Can you work these out from the drawing? Everything is in mm from the part's minimum corner. Round coordinates to 2 decimals unless told otherwise and drop trailing zeros. Order: outer loops, then holes, each group sorted by start corner. A loop starts at its lowest first (then second) coordinate and runs counter-clockwise, first axis right, second up. Notation, with made-up numbers: (-1.75, -39.75) -> (53.25, -39.75) arc R15 cw to (53.25, -11.75) -> close; hole circle Ø10 at (-18.75, 35.5). An arc over 180 degrees is marked (long way). One line per item, written item: value.
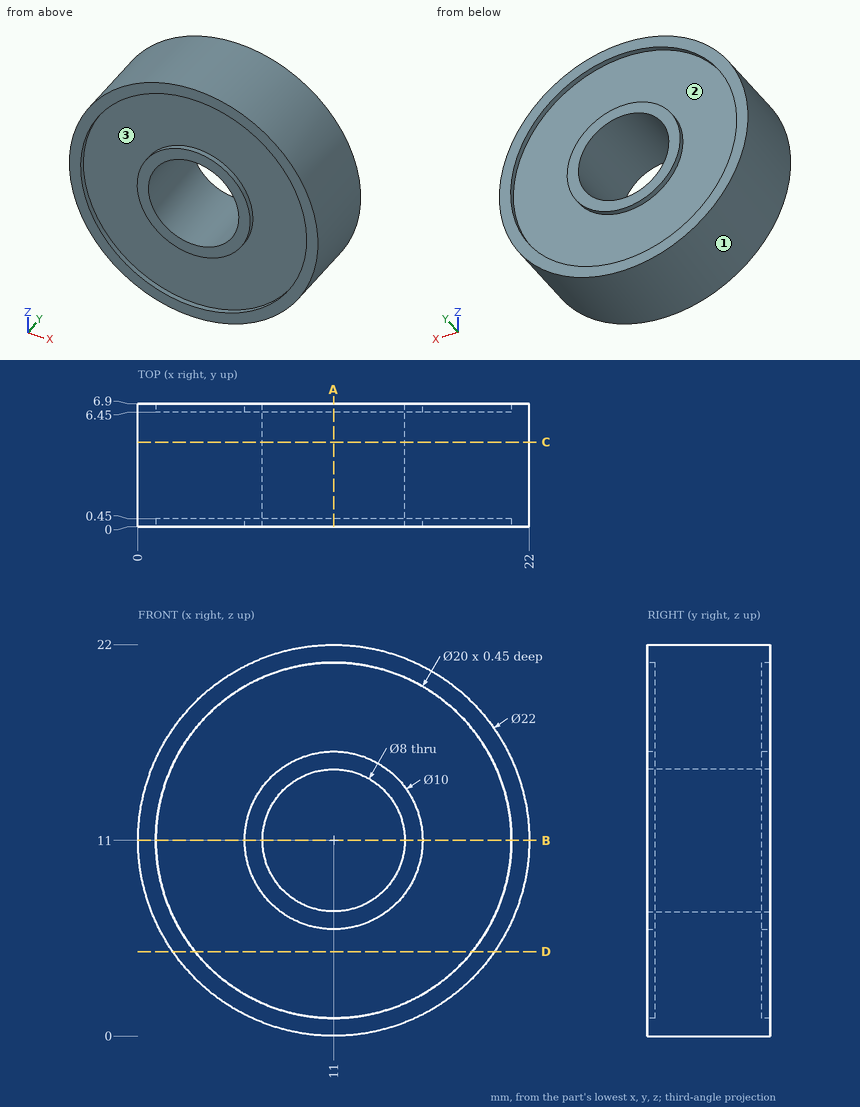
Q1. Will these pins go through, and if not, where does the flat tip stop? pin 1 Ø4 at (x, y) = (3, 4) entering from -Z; pin 2 Ø10 at (x, z) = (8.5, 6) entering from -Y; pin 3 Ø5 at (x, z) = (11, 11) entering from +Y.
Answers below:
pin 1: z = 1.78
pin 2: y = 0
pin 3: through
Q2. Please list where these lines run through material, in increasing order: line 1 along X through (y, z) = (6.6, 11); line 2 along X through (y, z) = (5.25, 11); line 3 along Y through (x, z) = (9, 3.25).
Answers below:
line 1: 0 to 1, 6 to 7, 15 to 16, 21 to 22
line 2: 0 to 7, 15 to 22
line 3: 0.45 to 6.45
Q3. I want a section at A-A on x = 11. List the corners of the cut face in (y, z) for me, plus the area to 3 significant figures.
Answers below:
outline: (0, 0) -> (6.9, 0) -> (6.9, 1) -> (6.45, 1) -> (6.45, 6) -> (6.9, 6) -> (6.9, 7) -> (0, 7) -> (0, 6) -> (0.45, 6) -> (0.45, 1) -> (0, 1) -> close; (0, 15) -> (6.9, 15) -> (6.9, 16) -> (6.45, 16) -> (6.45, 21) -> (6.9, 21) -> (6.9, 22) -> (0, 22) -> (0, 21) -> (0.45, 21) -> (0.45, 16) -> (0, 16) -> close
area: 87.6 mm^2
Q4. I want a section at D-D on z = 4.75. List the corners of the cut face in (x, y) for me, plus the area to 3 significant figures.
Answers below:
outline: (1.95, 0) -> (3.19, 0) -> (3.19, 0.45) -> (18.81, 0.45) -> (18.81, 0) -> (20.05, 0) -> (20.05, 6.9) -> (18.81, 6.9) -> (18.81, 6.45) -> (3.19, 6.45) -> (3.19, 6.9) -> (1.95, 6.9) -> close
area: 111 mm^2
Q5. I want a section at C-C on y = 4.75. List the corners of the cut face in (x, z) for me.
Answers below:
outline: circle Ø22 at (11, 11); hole circle Ø8 at (11, 11)
Q6. We'd pull the mould along X, two halves only. Please class the marked faces 1, 2 and 3: released by +X, released by -X, zero draft, split by the parting line, or undercut.
Answers below:
face 1: split by the parting line
face 2: undercut
face 3: undercut
Q7. I want a section at B-B on z = 11. List the corners of the cut face in (x, y) for me.
Answers below:
outline: (0, 0) -> (1, 0) -> (1, 0.45) -> (6, 0.45) -> (6, 0) -> (7, 0) -> (7, 6.9) -> (6, 6.9) -> (6, 6.45) -> (1, 6.45) -> (1, 6.9) -> (0, 6.9) -> close; (15, 0) -> (16, 0) -> (16, 0.45) -> (21, 0.45) -> (21, 0) -> (22, 0) -> (22, 6.9) -> (21, 6.9) -> (21, 6.45) -> (16, 6.45) -> (16, 6.9) -> (15, 6.9) -> close
